from build123d import *

# Parameters (mm, degrees)
F0_W     = 25.4
F0_H     = 57
F1_DEPTH = 2
F2_W     = 19.4
F2_H     = 9.1
F2_H_2   = 26.8
F3_DEPTH = 2.001
F4_R     = 7


with BuildPart() as f1:
    # F0 (on Top) → F1 (new body)
    with BuildSketch(Plane.XY):
        Rectangle(F0_W, F0_H)
    extrude(amount=F1_DEPTH)

    # F2 (on face) → F3 (cut, through all)
    with BuildSketch(Plane.XY.offset(2)):
        with Locations((0, 20.95)):
            Rectangle(F2_W, F2_H)
        Rectangle(F2_W, F2_H_2)
        with Locations((0, -20.95)):
            Rectangle(F2_W, F2_H)
    extrude(amount=-F3_DEPTH, mode=Mode.SUBTRACT)

    # F4
    f4_edges = [f1.edges().sort_by_distance(p)[0] for p in [
        (12.7, 28.5, 1),
        (12.7, -28.5, 1),
        (-12.7, -28.5, 1),
        (-12.7, 28.5, 1),
    ]]
    fillet(f4_edges, radius=F4_R)


solid = f1.part
The listing builds one solid part. Answer for the finished solid, in the listing's coordinates (mm). A direction names the side the tool comes from. Give positions to 0.01 mm unless a question says otherwise; leave off trailing zeros. Order: outer loops, then holes, each group sorted by start corner. A loop starts at its lowest first (then second) coordinate and runs counter-clockwise, first axis right, second up. Notation, with made-up numbers: (-35.5, 41.5) - (-6.5, 41.5) arc R6 ccw to (-6.5, 49.5) - close; hole circle Ø3 at (89.5, -1.75). An arc over 180 degrees is marked (long way). Answer as CSV lines item,"result".
Q1. Each of these flat-tipped pins is pushed along its axis until it touches: pin 1 Ø6 at (x, y) = (3, 17) entering from -Z; pin 2 Ø0.6 at (y, z) = (22.5, 0.5) entering from -X. Where does it stop, or does it pass through?
Answer key:
pin 1,"stops at z = 0"
pin 2,"stops at x = -12.66"
Q2. A cutting plane is placed at C-C, the plane z = 0.8. Determine the outline of the cut face in (x, y).
Answer key:
outline,"(-12.7, -21.5) arc R7 ccw to (-5.7, -28.5) - (5.7, -28.5) arc R7 ccw to (12.7, -21.5) - (12.7, 21.5) arc R7 ccw to (5.7, 28.5) - (-5.7, 28.5) arc R7 ccw to (-12.7, 21.5) - close; hole (-9.7, -25.5) - (9.7, -25.5) - (9.7, -16.4) - (-9.7, -16.4) - close; hole (-9.7, -13.4) - (9.7, -13.4) - (9.7, 13.4) - (-9.7, 13.4) - close; hole (-9.7, 16.4) - (9.7, 16.4) - (9.7, 25.5) - (-9.7, 25.5) - close"
Q3. A cutting plane is placed at D-D, the plane y = 22. Determine the outline of the cut face in (x, z), and give its area (3 significant figures).
Answer key:
outline,"(-12.68, 0) - (-9.7, 0) - (-9.7, 2) - (-12.68, 2) - close; (9.7, 0) - (12.68, 0) - (12.68, 2) - (9.7, 2) - close"
area,"11.9 mm^2"
Q4. Which of the six approach directions +Z, -Z, +X, -X, +Y, -Y give full straight-line access (tool end or side, diameter ignored) to faces 1 (the face through (-9.7, 21, 1)), 2 (the face through (-10.7, -26.4, 1))?
Answer key:
face 1,"+Z, -Z"
face 2,"+Z, -Z, -X, -Y"
Q5. A cutting plane is placed at B-B, the plane y = -4.5. Determine the outline of the cut face in (x, z).
Answer key:
outline,"(-12.7, 0) - (-9.7, 0) - (-9.7, 2) - (-12.7, 2) - close; (9.7, 0) - (12.7, 0) - (12.7, 2) - (9.7, 2) - close"
Q6. A cutting plane is placed at A-A, the plane x = -4. Determine the outline of the cut face in (y, z), and give its area (3 significant figures).
Answer key:
outline,"(-28.5, 0) - (-25.5, 0) - (-25.5, 2) - (-28.5, 2) - close; (-16.4, 0) - (-13.4, 0) - (-13.4, 2) - (-16.4, 2) - close; (13.4, 0) - (16.4, 0) - (16.4, 2) - (13.4, 2) - close; (25.5, 0) - (28.5, 0) - (28.5, 2) - (25.5, 2) - close"
area,"24.0 mm^2"
Q7. Straight lines are drawn through the part: L1, parallel to Y at x = -5.5, z = 1.8; L2, parallel to X at y = -13, z = 1.5; L3, parallel to Y at x = -9.5, z = 0.3. For each, find the intervals that lie inside material, in ascending order.
Answer key:
L1,"y = -28.5 to -25.5, -16.4 to -13.4, 13.4 to 16.4, 25.5 to 28.5"
L2,"x = -12.7 to -9.7, 9.7 to 12.7"
L3,"y = -27.38 to -25.5, -16.4 to -13.4, 13.4 to 16.4, 25.5 to 27.38"
Q8. Determine the mould class of faces 3 (the face through (0, 13.4, 1)), 4 (the face through (-10, 2, 0)), 5 (the face through (-10.7, 26.4, 1)) for opening direction Y: pulls with the +Y half, pulls with the -Y half, needs draft (parallel to the pull), parting line crosses it, or undercut.
Answer key:
face 3,"undercut"
face 4,"needs draft"
face 5,"pulls with the +Y half"
